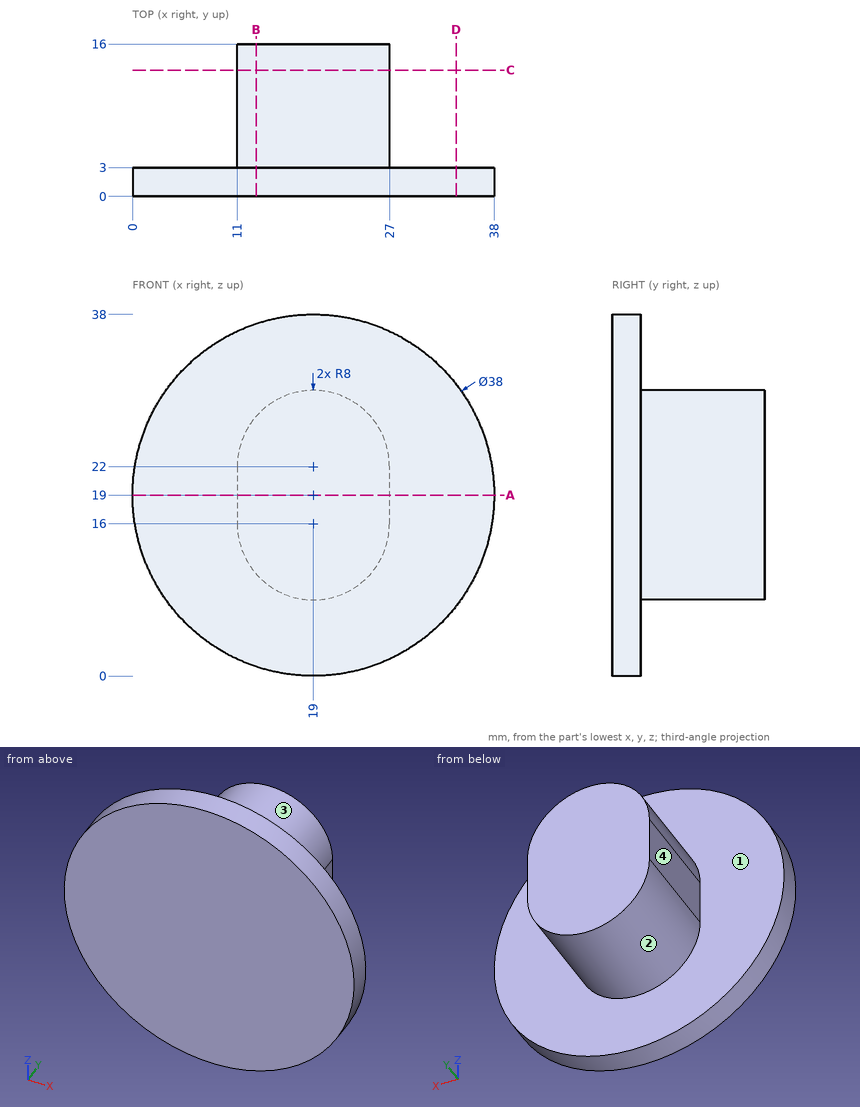
Answer from the drawing. Dimensions are ordinates in mm from the lowest x, y and z of the part. A direction names the side the tool comes from. Round coordinates to 2 decimals unless told otherwise and drop trailing zeros. Loops run counter-clockwise (first coordinate to the right, second up) from the corner with the lowest first, then second, coordinate; pieces in that order, holes last.
Q1. Each of these flat-tipped pins is pushed along its axis until it touches: pin 1 (8 mm diameter, centred on x = 4, z = 26.5, fed in from +Y); pin 2 (1 mm diameter, centred on y = 5, z = 27.5, fed in from -X) (3 decimals); pin 3 (8 mm diameter, centred on y = 7.5, z = 19, fed in from -X). Where does it stop, or does it pass through?
Q2. Section B-B on x = 13 is taken. Write down the section's boundary in (y, z).
Q3. Section C-C on y = 13.25 is taken. Write down the section's boundary in (x, z).
Q4. Section A-A on z = 19 is taken. Write down the section's boundary in (x, y), and give its area (3 significant figures).
Q5. Consider probe 1 along Y at (x, z) = (10, 10); probe 2 along Z at (x, y) = (19, 10.75); probe 3 along X at (y, z) = (11.5, 17). Determine where each line is inside the solid, lowest interval first.
Q6. Section D-D on x = 34 is taken. Write down the section's boundary in (y, z).
Q7. Which of the six approach directions +Z, -Z, +X, -X, +Y, -Y give full straight-line access (tool end or side, diameter ignored) to the marked faces 1, 2, 3 and 4?
Output:
1. pin 1: stops at y = 3
1. pin 2: stops at x = 12.755
1. pin 3: stops at x = 11
2. outline: (0, 0.97) - (3, 0.97) - (3, 10.71) - (16, 10.71) - (16, 27.29) - (3, 27.29) - (3, 37.03) - (0, 37.03) - close
3. outline: (11, 16) arc R8 ccw to (27, 16) - (27, 22) arc R8 ccw to (11, 22) - close
4. outline: (0, 0) - (38, 0) - (38, 3) - (27, 3) - (27, 16) - (11, 16) - (11, 3) - (0, 3) - close
4. area: 322 mm2
5. probe 1: y = 0 to 3
5. probe 2: z = 8 to 30
5. probe 3: x = 11 to 27
6. outline: (0, 7.34) - (3, 7.34) - (3, 30.66) - (0, 30.66) - close
7. face 1: +Y
7. face 2: -Z, +Y
7. face 3: +Z, +Y
7. face 4: +Z, -Z, -X, +Y
